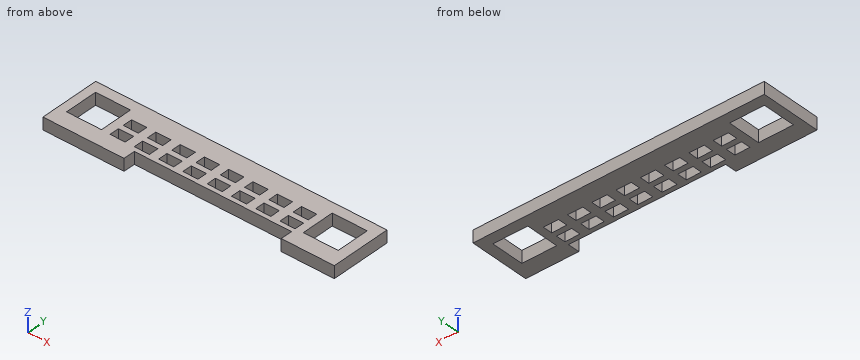
```python
from build123d import *

# Parameters (mm, degrees)
F0_W     = 96
F0_H     = 20
F2_DEPTH = 4
F1_W     = 11.5
F1_H     = 11
F1_W_2   = 5
F1_H_2   = 3.2
F1_W_3   = 51.8
F1_H_3   = 3.9
F3_DEPTH = 4.001


with BuildPart() as f2:
    # F0 (on Top) → F2 (new body)
    with BuildSketch(Plane.XY):
        with Locations((48, 10)):
            Rectangle(F0_W, F0_H)
    extrude(amount=F2_DEPTH)

    # F1 (on Top) → F3 (cut, through all)
    with BuildSketch(Plane.XY):
        with Locations((8.75, 11)):
            Rectangle(F1_W, F1_H)
        with Locations((86.75, 11)):
            Rectangle(F1_W, F1_H)
        with Locations((19.9, 12)):
            Rectangle(F1_W_2, F1_H_2)
        with Locations((19.9, 7)):
            Rectangle(F1_W_2, F1_H_2)
        with Locations((27.9, 12)):
            Rectangle(F1_W_2, F1_H_2)
        with Locations((27.9, 7)):
            Rectangle(F1_W_2, F1_H_2)
        with Locations((35.9, 12)):
            Rectangle(F1_W_2, F1_H_2)
        with Locations((35.9, 7)):
            Rectangle(F1_W_2, F1_H_2)
        with Locations((43.9, 12)):
            Rectangle(F1_W_2, F1_H_2)
        with Locations((43.9, 7)):
            Rectangle(F1_W_2, F1_H_2)
        with Locations((51.9, 12)):
            Rectangle(F1_W_2, F1_H_2)
        with Locations((51.9, 7)):
            Rectangle(F1_W_2, F1_H_2)
        with Locations((59.9, 12)):
            Rectangle(F1_W_2, F1_H_2)
        with Locations((59.9, 7)):
            Rectangle(F1_W_2, F1_H_2)
        with Locations((67.9, 12)):
            Rectangle(F1_W_2, F1_H_2)
        with Locations((67.9, 7)):
            Rectangle(F1_W_2, F1_H_2)
        with Locations((75.9, 12)):
            Rectangle(F1_W_2, F1_H_2)
        with Locations((75.9, 7)):
            Rectangle(F1_W_2, F1_H_2)
        with Locations((52.6, 1.95)):
            Rectangle(F1_W_3, F1_H_3)
    extrude(amount=F3_DEPTH, mode=Mode.SUBTRACT)


solid = f2.part
```
CAD build for the part. Positions are in the model's coordinates, mm. Coordinates: 2 decimals unless noted, no trailing zeros. Write each loop counter-clockwise with the first axis right and the second up, starting at its lowest first coordinate (ties: lowest second). Pieces come first, ordered by that corner, then holes.
(1) Cut at B-B, the plane x = 19. List the corners of the cut face in (y, z), and give its area (3 significant figures).
(2) Cut at D-D, the plane y = 6.75. Count the separate pieces of the cut face and the enclosed holes in it, and give its area (3 significant figures).
(3) Cut at C-C, the plane x = 9. List the corners of the cut face in (y, z), and give its area (3 significant figures).
(4) Cut at A-A, the plane y = 1.5. List the corners of the cut face in (x, z), and give its area (3 significant figures).
(5) Drill centre lines: probe 1 along Y at (x, z) = (34, 0.6); probe 2 along X at (y, z) = (10, 3); probe 3 along Y at (x, z) = (19.5, 1.8). Where is each one in solid material? Low to high.
(6) Flat gauge pin, fed straight in: pin 1 (2 mm diameter, centred on x = 52, z = 3, fed in from -Y). Where does the tip first touch, or does it go through?
Geometry says:
1. outline: (0, 0) - (5.4, 0) - (5.4, 4) - (0, 4) - close; (8.6, 0) - (10.4, 0) - (10.4, 4) - (8.6, 4) - close; (13.6, 0) - (20, 0) - (20, 4) - (13.6, 4) - close
1. area: 54.4 mm2
2. separate pieces: 11
2. enclosed holes: 0
2. area: 132 mm2
3. outline: (0, 0) - (5.5, 0) - (5.5, 4) - (0, 4) - close; (16.5, 0) - (20, 0) - (20, 4) - (16.5, 4) - close
3. area: 36.0 mm2
4. outline: (0, 0) - (26.7, 0) - (26.7, 4) - (0, 4) - close; (78.5, 0) - (96, 0) - (96, 4) - (78.5, 4) - close
4. area: 177 mm2
5. probe 1: y = 3.9 to 5.4, 8.6 to 10.4, 13.6 to 20
5. probe 2: x = 0 to 3, 14.5 to 81, 92.5 to 96
5. probe 3: y = 0 to 5.4, 8.6 to 10.4, 13.6 to 20
6. pin 1: stops at y = 3.9
